Input: part model. Units: mm. Frame: model coordinates. A direction names the side the tool comes from. Round coordinates to 2 decimals unless told otherwise and drop trailing zeros. Order: outer loops, then holes, each group sorted by start corner. A loop starts at its lowest first (then second) coordinate and runs counter-clockwise, first axis right, second up. Notation, with made-up numbers: (-22, -33) -> (35, -33) arc R17 cw to (35, -16) -> close; hole circle Ø2 at (-31.5, -25). An arc over 180 degrees is marked (long way). Answer as CSV lines item,"result". Start each with the question number.
1) Access query for faces 4 (the face through (-0.28, 1.57, 47.22)), 5 (the face through (-104.118, 1.565, 6.386)), 6 (the face through (-29.52, 1.57, 37.74)). Directions: +Z, -Z, +X, -X, +Y, -Y. A direction counts if a zero-diameter tool reaches every point of the face in a straight line with its end or side. Return the directions, or none.
2) Section query B-B, the plane z = 26. Output: boundary loops of the cut face in (x, y) (3 decimals).
3) Section query D-D, the plane z = 57. Output: boundary loops of the cut face in (x, y) (3 decimals), and give its area (3 significant figures).
4) Mould query, pull axis Z, two halves, no side actions, for faces 1 (the face through (-64.41, 1.565, 40.243)), 2 (the face through (-8.793, 1.565, 10.836)), 3 (the face through (-47, 3.175, 19)). Classes: +Z half, -Z half, draft (parallel to the pull), parting line (faces both ways), or undercut.
5) Section query C-C, the plane y = 2.65. Output: boundary loops of the cut face in (x, z) (1 decimal), and give its area (3 significant figures).
6) First-contact query: P1, Ø1.5, axis at y = 1.5, z = 47, coming from the +X side. Flat tip, straight axial feed; report the tip coordinate or a pass-through.
7) Section query A-A, the plane x = -8.5. Output: boundary loops of the cut face in (y, z) (3 decimals).
8) Line query: L1, parallel to X at y = 2.5, z = 15; L2, parallel to Z at x = -88, y = 0.3; L3, parallel to Z at x = 5.5, y = 2.55. Output: solid intervals per line, ascending.
Autodesk Inventor part; units mm, degrees
ref_plane "YZ Plane" through (0, 0, 0) normal (1, 0, 0) x (0, 1, 0)
ref_plane "XZ Plane" through (0, 0, 0) normal (0, 1, 0) x (-1, 0, 0)
ref_plane "XY Plane" through (0, 0, 0) normal (0, 0, 1) x (1, 0, 0)
sketch "Sketch1" plane through (0, 0, 0) normal (0, 1, 0) x (-1, 0, 0)
  line L0 (103.4591, 16.4441) -> (104.7625, 17.6511)
  arc A0 (104.7625, 17.6511) -> (105.6235, 20.966) centre (102.6053, 19.9807) ccw
  line L1 (105.6235, 20.966) -> (100.9494, 35.2839)
  arc A1 (100.9494, 35.2839) -> (87.8224, 43.4902) centre (89.4801, 31.5396) ccw
  line L2 (87.8224, 43.4902) -> (40.332, 36.9027)
  arc A2 (19.8124, 43.2164) -> (40.332, 36.9027) centre (36.8421, 62.0618) ccw
  line L3 (19.8124, 43.2164) -> (-6.8947, 67.3504)
  arc A3 (-6.8947, 67.3504) -> (-9.362, 65.4298) centre (-7.959, 66.1726) ccw
  line L4 (-9.362, 65.4298) -> (10.1942, 28.4903)
  arc A4 (-8.303, 4.7241) -> (10.1942, 28.4903) centre (-4.3971, 20.7654) ccw
  arc A5 (-8.303, 4.7241) -> (-9.218, 2.3787) centre (-8.6034, 3.4901) ccw
  arc A6 (-9.218, 2.3787) -> (0, 0) centre (0, 19.05) ccw
  line L5 (0, 0) -> (102.7651, 0)
  arc A7 (102.7651, 0) -> (105.0946, 5.3323) centre (102.7651, 3.175) ccw
  line L6 (105.0946, 5.3323) -> (103.1146, 7.4705)
  arc A8 (103.4591, 16.4441) -> (103.1146, 7.4705) centre (107.7737, 11.785) ccw
  circle A9 centre (89.4801, 31.5396) radius 6.985
  circle A10 centre (21.1327, 13.2882) radius 2.2479
  circle A11 centre (59.2327, 13.2882) radius 2.2479
  point P0 (0, 0)
  point P1 (-8.303, 4.7241)
  point P2 (-9.218, 2.3787)
  point P3 (0, 0)
  point P4 (102.7651, 0)
  point P5 (105.0946, 5.3323)
  point P6 (105.6235, 20.966)
  point P7 (19.8124, 43.2164)
  point P8 (-9.362, 65.4298)
  point P9 (10.1942, 28.4903)
extrude "Plate1" add sketch "Sketch1" along normal blind 3.175
equation "\"d0\" = Thickness"
equation "\"BendRadius\" = Thickness"
equation "\"BendReliefWidth\" = Thickness"
equation "\"BendReliefDepth\" = 0.5 * Thickness"
equation "\"CornerReliefSize\" = 4 * Thickness"
equation "\"MinimumRemnant\" = 2 * Thickness"
equation "\"TransitionRadius\" = BendRadius"
equation "\"JacobiRadiusSize\" = BendRadius"
equation "\"GapSize\" = Thickness"
properties part number "hook-top-plate" material "Aluminum 6061"
Findings:
1,face 4,"+X, +Y, -Y"
1,face 5,"-X, +Y, -Y"
1,face 6,"+Z, +Y, -Y"
2,outline,"(-103.98, 0) -> (-93.735, 0) -> (-93.735, 3.175) -> (-103.98, 3.175) -> close; (-85.225, 0) -> (-11.261, 0) -> (-11.261, 3.175) -> (-85.225, 3.175) -> close"
3,outline,"(-4.559, 0) -> (4.899, 0) -> (4.899, 3.175) -> (-4.559, 3.175) -> close"
3,area,"30.0 mm^2"
4,face 1,"+Z half"
4,face 2,"undercut"
4,face 3,"draft"
5,outline,"(-105.6, 21) arc R3.2 ccw to (-104.8, 17.7) -> (-103.5, 16.4) arc R6.3 cw to (-103.1, 7.5) -> (-105.1, 5.3) arc R3.2 ccw to (-102.8, 0) -> (0, 0) arc R19 ccw to (9.2, 2.4) arc R1.3 ccw to (8.3, 4.7) arc R16.5 cw to (-10.2, 28.5) -> (9.4, 65.4) arc R1.6 ccw to (6.9, 67.4) -> (-19.8, 43.2) arc R25.4 cw to (-40.3, 36.9) -> (-87.8, 43.5) arc R12.1 ccw to (-100.9, 35.3) -> close; hole circle Ø14 at (-89.5, 31.5); hole circle Ø4.5 at (-59.2, 13.3); hole circle Ø4.5 at (-21.1, 13.3)"
5,area,"3,970 mm^2"
6,P1,"stops at x = 0"
7,outline,"(0, 0) -> (3.175, 0) -> (3.175, 10.458) -> (0, 10.458) -> close; (0, 31.69) -> (3.175, 31.69) -> (3.175, 53.439) -> (0, 53.439) -> close"
8,L1,"x = -102.3 to -60.69, -57.78 to -22.59, -19.68 to -11.07"
8,L2,"z = 0 to 24.71, 38.37 to 43.51"
8,L3,"z = 0.81 to 4.29, 58.13 to 66.09"
